from build123d import *

# Parameters (mm, degrees)
SKETCH1_R               = 20.25
SKETCH1_R_2             = 3.682229715
BOSS_EXTRUDE1_DEPTH     = 15
SKETCH2_R               = 20.25
BOSS_EXTRUDE2_DEPTH     = 3
SKETCH3_W               = 2.140111698
SKETCH3_H               = 9.021804968
CUT_EXTRUDE1_DEPTH      = 13
CUT_EXTRUDE1_DEPTH_BACK = 4


with BuildPart() as part:
    # Sketch1 → Boss-Extrude1 (new body)
    with BuildSketch(Plane(origin=(0, 0, 0), x_dir=(1, 0, 0), z_dir=(0, 1, 0))):
        with BuildLine():
            Line((-25.477303851, -15.433164228), (-25.477303851, 15.022696149))
            ThreePointArc((-25.477303851, 15.022696149), (-25.477303851, 25.477303851), (-15.022696149, 25.477303851))
            Line((-15.022696149, 25.477303851), (15.433164228, 25.477303851))
            ThreePointArc((15.433164228, 25.477303851), (25.887771929, 25.477303851), (25.887771929, 15.022696149))
            Line((25.887771929, 15.022696149), (25.887771929, -15.433164228))
            ThreePointArc((25.887771929, -15.433164228), (25.887771929, -25.887771929), (15.433164228, -25.887771929))
            Line((15.433164228, -25.887771929), (-15.022696149, -25.887771929))
            ThreePointArc((-15.022696149, -25.887771929), (-25.477303851, -25.887771929), (-25.477303851, -15.433164228))
        make_face()
        Circle(SKETCH1_R, mode=Mode.SUBTRACT)
        with Locations((-20.25, 20.25)):
            Circle(SKETCH1_R_2, mode=Mode.SUBTRACT)
        with Locations((20.25, 20.25)):
            Circle(SKETCH1_R_2, mode=Mode.SUBTRACT)
        with Locations((20.25, -20.25)):
            Circle(SKETCH1_R_2, mode=Mode.SUBTRACT)
        with Locations((-20.25, -20.25)):
            Circle(SKETCH1_R_2, mode=Mode.SUBTRACT)
    extrude(amount=BOSS_EXTRUDE1_DEPTH)

    # Sketch2 → Boss-Extrude2 (add)
    with BuildSketch(Plane.XZ):
        Circle(SKETCH2_R)
    extrude(amount=-BOSS_EXTRUDE2_DEPTH)

    # Sketch3 → Cut-Extrude1 (cut, two sides)
    with BuildSketch(Plane(origin=(0, 3, 0), x_dir=(1, 0, 0), z_dir=(0, 1, 0))) as cut_extrude1_sk:
        with Locations((20.25, 0)):
            Rectangle(SKETCH3_W, SKETCH3_H)
    extrude(amount=CUT_EXTRUDE1_DEPTH, mode=Mode.SUBTRACT)
    extrude(cut_extrude1_sk.sketch, amount=-CUT_EXTRUDE1_DEPTH_BACK, mode=Mode.SUBTRACT)


solid = part.part
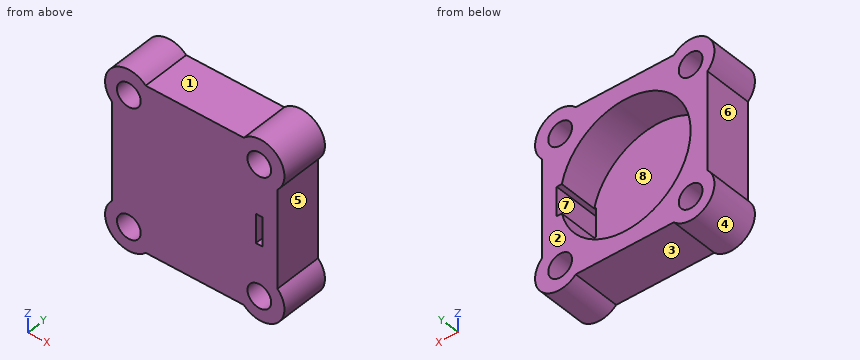
Verification items for the finished model (mm, model axes). Face numbers are marked on the shaded views. A direction names the side the tool comes from. Coordinates: 2 decimals unless noted, no trailing zeros. Order: outer loops, then holes, each group sorted by start corner. A loop starts at its lowest first (then second) coordinate and runs counter-clockwise, first axis right, second up.
Item 1: Depth check by flat-ended pin: pin 1 (12 mm diameter, centred on x = 8, z = -10.5, fed in from -Y); pin 2 (6 mm diameter, centred on y = 7, z = -11.5, fed in from +X); pin 3 (20 mm diameter, centred on x = 3.5, z = -2.5, fed in from +Y); pin 4 (7 mm diameter, centred on y = 10, z = 1, fed in from -X). Enter the tip coordinate at first touch or a pass-through.
Filled in:
pin 1: stops at y = 0
pin 2: stops at x = 25.89
pin 3: stops at y = 3
pin 4: stops at x = -25.48
Item 2: Material ranges on L1, parallel to X at y = 3.25, z = 20.5; L2, parallel to Z at x = 20.25, y = 4.25; L3, parallel to Z at x = -22, y = 10, recorded low to high.
Filled in:
L1: x = -27.64 to -23.92, -16.58 to 16.58, 23.92 to 28.05
L2: z = -27.63 to -23.93, -16.57 to -4.51, 4.51 to 16.57, 23.93 to 28.04
L3: z = -27.43 to -23.49, -17.01 to 17.01, 23.49 to 27.84
Item 3: Section check A-A, the plane y = 10.5. Enter the section's corners in (x, z), then the cut area to 3 significant figures.
Filled in:
outline: (-25.48, -15.02) arc R7.39 ccw to (-15.02, -25.48) - (15.43, -25.48) arc R7.39 ccw to (25.89, -15.02) - (25.89, 15.43) arc R7.39 ccw to (15.43, 25.89) - (-15.02, 25.89) arc R7.39 ccw to (-25.48, 15.43) - close; hole circle Ø7.36 at (-20.25, -20.25); hole circle Ø7.36 at (-20.25, 20.25); hole circle Ø7.36 at (20.25, -20.25); hole circle Ø7.36 at (20.25, 20.25); hole (19.74, -4.51) - (21.32, -4.51) - (21.32, 4.51) - (19.74, 4.51) arc R20.25 ccw (long way) to start
area: 1,290 mm2
Item 4: Section check C-C, the plane z = 22. Enter the section's corners in (x, y), then the cut area to 3 significant figures.
Filled in:
outline: (-27.52, 0) - (-23.49, 0) - (-23.49, 15) - (-27.52, 15) - close; (-17.01, 0) - (17.01, 0) - (17.01, 15) - (-17.01, 15) - close; (23.49, 0) - (27.93, 0) - (27.93, 15) - (23.49, 15) - close
area: 637 mm2
Item 5: Access from +Z, -Z, +X, -X, +Y, -Y to the whole of each face (thin tool, end or side, straight path). Record for the marked faces 5, 6, 7 and 8.
Filled in:
face 5: +X, +Y, -Y
face 6: -X, +Y, -Y
face 7: +Y, -Y
face 8: +Y
Item 6: Release check for a two-part mould opening along Z. For the marked faces 1, 2, 3 and 4 record: +Z half, -Z half, draft (parallel to the pull), parting line (faces both ways), or undercut.
Filled in:
face 1: +Z half
face 2: draft
face 3: -Z half
face 4: undercut
Item 7: Section check B-B, the plane x = 0. Enter the section's corners in (y, z), then the cut area to 3 significant figures.
Filled in:
outline: (0, -25.48) - (15, -25.48) - (15, -20.25) - (3, -20.25) - (3, 20.25) - (15, 20.25) - (15, 25.89) - (0, 25.89) - close
area: 284 mm2
Item 8: Section check D-D, the plane x = 22. Enter the section's corners in (y, z).
Filled in:
outline: (0, -27.52) - (15, -27.52) - (15, -23.49) - (0, -23.49) - close; (0, -17.01) - (15, -17.01) - (15, 17.01) - (0, 17.01) - close; (0, 23.49) - (15, 23.49) - (15, 27.93) - (0, 27.93) - close
